Can you work these out from the model? Positions are in its coordinate system, mm. Face numbers are marked on the shaded views. A direction names the side the tool comes from. Coordinates: 2 decimals unless noted, no trailing zeros. Order: outer loops, then holes, each group sorted by start corner. A loop starts at its lowest first (then second) coordinate and runs counter-clockwise, first axis right, second up. Notation, with made-up numbers: M 55.25,-16.75 L 72.25,-16.75 A22 cw 72.25,-9.75 Z; hole C 16.5,51 d8. An arc over 180 degrees is marked long. Answer as a JSON object with one key per item and string values.
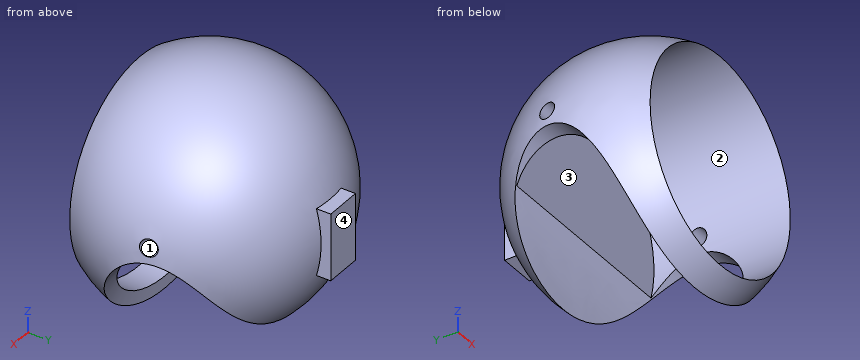
from build123d import *

# Parameters (mm, degrees)
CUT_EXTRUDE2_DEPTH      = 40
CUT_EXTRUDE2_DEPTH_BACK = 75
SKETCH2_R               = 62.5
CUT_EXTRUDE4_DEPTH      = 130.903810568
CUT_EXTRUDE4_DEPTH_BACK = 130.903810568
SKETCH6_W               = 22
SKETCH6_H               = 40
BOSS_EXTRUDE1_DEPTH     = 5
CUT_EXTRUDE5_DEPTH      = 133.853302556
CUT_EXTRUDE5_DEPTH_BACK = 133.853302556
SKETCH8_R               = 5


with BuildPart() as part:
    # Sketch1 → Revolve1 (revolve)
    with BuildSketch(Plane.XY):
        with BuildLine():
            Line((0, 75), (0, -75))
            ThreePointArc((0, -75), (-75, 0), (0, 75))
        make_face()
    revolve(axis=Axis((0, 124.688842105, 0), (0, -1, 0)))

    # Sketch2 → Cut-Extrude2 (cut, two sides: drawn at the far end of the back side and taken through both)
    with BuildSketch(Plane(origin=(0, 0, 0), x_dir=(1, 0, 0), z_dir=(0, 1, 0)).offset(-CUT_EXTRUDE2_DEPTH_BACK)):
        with Locations(Location((0, 0, 0), (0, 0, 270))):
            Circle(SKETCH2_R)
    extrude(amount=CUT_EXTRUDE2_DEPTH + CUT_EXTRUDE2_DEPTH_BACK, mode=Mode.SUBTRACT)

    # Sketch3 → Cut-Extrude4 (cut, two sides: drawn at the far end of the back side and taken through both)
    with BuildSketch(Plane(origin=(0, 0, 0), x_dir=(0, 0, -1), z_dir=(1, 0, 0)).offset(-CUT_EXTRUDE4_DEPTH_BACK)):
        with BuildLine():
            ThreePointArc((70.281956591, -26.181034696), (73.381820705, 15.495431263), (53.696962514, 52.360636137))
            add(Edge.make_bspline(
                [(53.696962514, 52.360636137), (-6.667727446, 43.107629562), (0.48026113, 9.256850763), (7.628249706, -24.593928036), (70.281956591, -26.181034696)],
                knots=[4.987408854, 4.987408854, 4.987408854, 6.397396854, 6.397396854, 7.807384853, 7.807384853, 7.807384853], degree=2, weights=[1, 0.76161544, 1, 0.76161544, 1]))
        make_face()
    extrude(amount=CUT_EXTRUDE4_DEPTH + CUT_EXTRUDE4_DEPTH_BACK, mode=Mode.SUBTRACT)

    # Sketch6 → Boss-Extrude1 (add, symmetric)
    with BuildSketch(Plane(origin=(0, 75, 0), x_dir=(1, 0, 0), z_dir=(0, 1, 0))):
        Rectangle(SKETCH6_W, SKETCH6_H)
    extrude(amount=BOSS_EXTRUDE1_DEPTH, both=True)

    # Sketch8 → Cut-Extrude5 (cut, two sides: drawn at the far end of the back side and taken through both)
    with BuildSketch(Plane(origin=(0, 0, 0), x_dir=(0, 0, -1), z_dir=(1, 0, 0)).offset(-CUT_EXTRUDE5_DEPTH_BACK)):
        with Locations((-9.331175984, 12.950127065)):
            Circle(SKETCH8_R)
    extrude(amount=CUT_EXTRUDE5_DEPTH + CUT_EXTRUDE5_DEPTH_BACK, mode=Mode.SUBTRACT)


solid = part.part
Item 1: I want a section at A-A, the plane y = 64. Write out the boundary of the cut face in (x, z).
Answers follow:
{"outline": "C 0,0 d78.2"}
Item 2: If we mould it in two halves opening along X, with no side actions, what happens to the marked faces 3 and 4? For each: pulls with the +X half, pulls with the -X half, needs draft (parallel to the pull), parting line crosses it, or undercut.
Answers follow:
{"face 3": "undercut", "face 4": "needs draft"}
Item 3: I'm going to push flat-ended pins straight in: pin 1 (1.5 mm diameter, centred on x = 41, y = -5, fed in from +Z); pin 2 (12 mm diameter, centred on y = 20.5, z = 18.5, fed in from -X); pin 3 (1 mm diameter, centred on y = 10.5, z = 18, fed in from -X). Where does each tip first touch, or does it pass through?
Answers follow:
{"pin 1": "stops at z = 63.09", "pin 2": "stops at x = -71.82", "pin 3": "stops at x = -72.19"}
Item 4: Which directions (+Z, -Z, +X, -X, +Y, -Y) give clear straight access to the entire face, cutting with the end or side of a thin tool? Please do the marked faces 1 and 2.
Answers follow:
{"face 1": "+X, -X", "face 2": "-Y"}
Item 5: I want a section at B-B, the plane z = 44. Write out the boundary of the cut face in (x, y).
Answers follow:
{"outline": "M -44.39,-41.46 L -44.39,40 L 44.39,40 L 44.39,-41.46 A60.74 ccw long Z"}
Item 6: Please list where these lines run through material, in increasing order: line 1 (X direction, y = 4, z = 0); line 2 (X direction, y = 23, z = 34); line 3 (Z direction, x = -38, y = -31).
Answers follow:
{"line 1": "x = -74.89 to -62.5, 62.5 to 74.89", "line 2": "x = -62.77 to -52.44, 52.44 to 62.77", "line 3": "z = -56.75 to -49.62, 49.62 to 56.75"}
